Input: part model. Units: mm. Frame: model coordinates. A direction names the side the tool comes from. Round coordinates to 2 decimals unless told otherwise and drop trailing zeros. Loops run counter-clockwise (first coordinate to the right, second up) from the corner with the lowest first, then second, coordinate; pieces in that order, holes last. Notation, with made-up numbers: M 78.25,19 L 135.25,19 A23 ccw 135.25,57 Z; hole C 75,88 d8. An arc over 180 degrees is marked long. Use one line per item in the form item = value. Start each with the question number.
Q1. Ray query, line 1 along Y through (x, z) = (6.5, 7.75); line 2 along X through (y, z) = (0, 7.5); line 3 along Y through (x, z) = (16.5, 7). Return the intervals inside material, ascending.
Q2. First-contact query: P1, Ø5, axis at y = -4, z = 7, coming from the +X side; P2, Ø6, axis at x = 14.5, z = 8, coming from the +Y side; P3, Ø2, axis at x = 11.5, y = -8.5, coming from the +Z side. Flat tips, straight axial feed; report the tip coordinate or a pass-through.
Q3. Section query B-B, the plane x = 6. Output: boundary loops of the cut face in (y, z).
Q4. Section query A-A, the plane z = 6.5. Output: boundary loops of the cut face in (x, y), and give its area (3 significant figures).
Q5. Section query C-C, the plane y = 9. Output: boundary loops of the cut face in (x, z).
Q6. Section query D-D, the plane x = 18.5. Output: boundary loops of the cut face in (y, z), and give its area (3 significant figures).
Q7. Access query for faces 5 (the flat face through (-4.1, -11.5, 10)), 6 (the cylindrical face through (19.43, 14.4, 4.06)), 7 (the flat face through (0, 11, 5)), 8 (the flat face through (-20, 0, 4)). Directions: +Z, -Z, +X, -X, +Y, -Y. A direction counts if a zero-diameter tool reaches every point of the face in a straight line with its end or side. Return the directions, or none.
Q8. Mould query, pull axis Y, two halves, no side actions, for faces 1 (the cylindrical face through (19.4, -14.43, 4.06)), 2 (the flat face through (16, 0, 5)), 3 (the flat face through (-23, 0, -1)), 4 (the flat face through (0, 15, 4)). Classes: pulls with the +Y half, pulls with the -Y half, needs draft (parallel to the pull), parting line crosses it, or undercut.
```python
from build123d import *

# Parameters (mm, degrees)
F0_W     = 40
F0_H     = 30
F0_W_2   = 32
F0_H_2   = 22
F1_DEPTH = 10
F0_W_3   = 46
F0_H_3   = 36
F2_DEPTH = 3
F3_R     = 2


with BuildPart() as f1:
    # F0 (on Top) → F1 (new body)
    with BuildSketch(Plane.XY):
        Rectangle(F0_W, F0_H)
        Rectangle(F0_W_2, F0_H_2, mode=Mode.SUBTRACT)
    extrude(amount=F1_DEPTH)

    # F0 (on Top) → F2 (join)
    with BuildSketch(Plane.XY):
        Rectangle(F0_W_3, F0_H_3)
        Rectangle(F0_W, F0_H, mode=Mode.SUBTRACT)
        Rectangle(F0_W, F0_H)
        Rectangle(F0_W_2, F0_H_2, mode=Mode.SUBTRACT)
        Rectangle(F0_W_2, F0_H_2)
    extrude(amount=-F2_DEPTH)

    # F3
    f3_edges = [f1.edges().sort_by_distance(p)[0] for p in [
        (-20, -15, 5),
        (-20, 15, 5),
        (20, -15, 5),
        (0, -15, 10),
        (-20, 0, 10),
        (0, 15, 10),
        (20, 0, 10),
        (20, 15, 5),
        (23, 18, -1.5),
        (23, -18, -1.5),
        (-23, -18, -1.5),
        (-23, 18, -1.5),
    ]]
    fillet(f3_edges, radius=F3_R)


solid = f1.part
```
Results found:
q1.line_1 = -15 to -11, 11 to 15
q1.line_2 = -20 to -16, 16 to 20
q1.line_3 = -15 to 15
q2.P1 = 20
q2.P2 = 15
q2.P3 = 0
q3.outline = M -18,-3 L 18,-3 L 18,0 L 15,0 L 15,8 A2 ccw 13,10 L 11,10 L 11,0 L -11,0 L -11,10 L -13,10 A2 ccw -15,8 L -15,0 L -18,0 Z
q4.outline = M -20,-13 A2 ccw -18,-15 L 18,-15 A2 ccw 20,-13 L 20,13 A2 ccw 18,15 L -18,15 A2 ccw -20,13 Z; hole M -16,-11 L 16,-11 L 16,11 L -16,11 Z
q4.area = 493 mm²
q5.outline = M -23,-3 L 23,-3 L 23,0 L 20,0 L 20,8 A2 ccw 18,10 L 16,10 L 16,0 L -16,0 L -16,10 L -18,10 A2 ccw -20,8 L -20,0 L -23,0 Z
q6.outline = M -18,-3 L 18,-3 L 18,0 L 14.94,0 L 14.94,8 A1.94 ccw 13,9.94 L -13,9.94 A1.94 ccw -14.94,8 L -14.94,0 L -18,0 Z
q6.area = 403 mm²
q7.face_5 = +Z, +X, -X, +Y, -Y
q7.face_6 = +Z, +X, +Y
q7.face_7 = +Z
q7.face_8 = +Z, -X, +Y, -Y
q8.face_1 = pulls with the -Y half
q8.face_2 = undercut
q8.face_3 = needs draft
q8.face_4 = pulls with the +Y half
